Part model, mm, in its own coordinate system. Face numbers are marked on the shaded views. A direction names the side the tool comes from. Give positions to 0.01 mm unless a question says otherwise; leave off trailing zeros. Write each loop counter-clockwise with the first axis right and the second up, starting at its lowest first coordinate (ties: lowest second). Pieces come first, ordered by that corner, then holes.
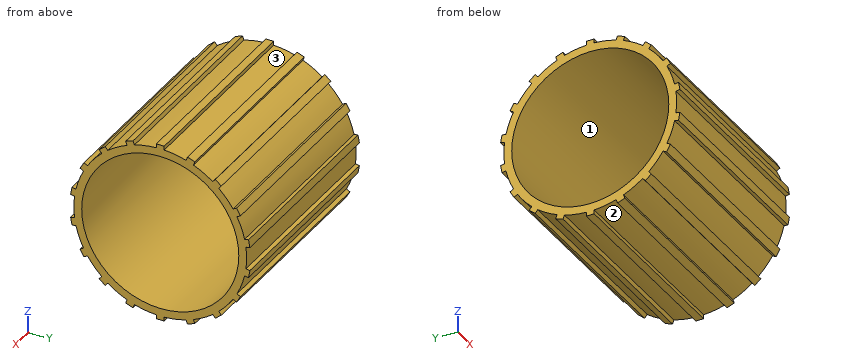
Autodesk Fusion 360 part; units mm, degrees
sketch "Sketch1" plane through (0, 0, 0) normal (0, 1, 0) x (1, 0, 0) in component "tread"
  line L0 (-50, 22) -> (0, 22)
  line L1 (0, 22) -> (0, 20)
  line L2 (0, 20) -> (-50, 20)
  line L3 (-50, 20) -> (-50, 22)
  line L4 (0, 0) -> (0, -12) construction
  dimension "d1" = 50
  dimension "d2" = 2
  dimension "d3" = 20
revolve "Revolve1" add sketch "Sketch1" angle 360 about axis through (1.75, 0, 0) along (1, 0, 0) makes body 1 in component "tread"
sketch "Sketch2" plane through (0, 0, 0) normal (0, 0, 1) x (1, 0, 0) in component "tread"
  line L0 (0, 0) -> (-50, 0)
  line L1 (0, 1) -> (-50, 1)
  line L2 (0, -1) -> (-50, -1)
  line L3 (0, -1) -> (0, 1)
  line L4 (-50, -1) -> (-50, 1)
  dimension "d5" = 50
  dimension "d6" = 1
  dimension "d7" = -1
extrude "Extrude1" add sketch "Sketch2" along normal mid plane 46 separate body makes body 2 in component "tread"
pattern_circular "C-Pattern1" count 9 over 360 about axis through (1.75, 0, 0) along (1, 0, 0) of "Extrude1" makes body 3 makes body 4 makes body 5 makes body 6 makes body 7 makes body 8 makes body 9 makes body 10 in component "tread"
sketch "Sketch3" plane through (0, 0, 0) normal (1, 0, 0) x (0, 0, -1) in component "tread"
  circle A0 centre (0, 0) radius 20
  dimension "d14" = 40
extrude "Extrude2" cut sketch "Sketch3" against normal blind 50 bodies 2 makes body 11 at (-16.6667, 1, -20.9833) in component "tread"
extrude "Extrude3" cut sketch "Sketch3" against normal blind 50 bodies 3 4 5 6 7 8 9 10 makes body 19 at (-16.6667, -13.3699, -17.4894) makes body 18 at (-33.3333, -20.4909, -4.6285) makes body 17 at (-33.3333, -18.6721, 9.6256) makes body 16 at (-16.6667, -8.4613, 20.3234) makes body 15 at (-16.6667, 6.5819, 21.0074) makes body 14 at (-16.6667, 18.5453, 11.8619) makes body 13 at (-16.6667, 21.8312, -2.834) makes body 12 at (-16.6667, 14.902, -16.2038) in component "tread"
combine "Combine1" operation add target body 1 tool bodies 5 in component "tread"
combine "Combine2" operation add target body 1 tool bodies 3 4 8 6 7 9 10 13 12 11 18 19 2 16 15 14 17 in component "tread"
component "tread" placed x (1, 0, 0) y (0, 1, 0) z (0, 0, 1) at (0, 0, 0)
1) 3-axis set-ups, long thin cutter, end or side, ignore diameter. For the marked faces 1, 2 and 3: which of +Z, -Z, +X, -X, +Y, -Y reach the whole face in a straight line?
Answers follow:
face 1: +X, -X
face 2: -Z, +X, -X
face 3: +Z, +X, -X
2) Wall check: L1, parallel to Y at x = -39, z = 0; L2, parallel to Z at x = -11, y = 0; L3, parallel to Y at x = -35.5, z = 8.5. Give the ranges that are in metal, low to high.
Answers follow:
L1: y = -22 to -20, 20 to 22
L2: z = -23 to -20, 20 to 23
L3: y = -20.29 to -18.1, 18.1 to 20.29
3) Pin check, flat tips, straight feed: pin 1 Ø1.5 at (x, z) = (-32, 4.5) entering from +Y; pin 2 Ø0.8 at (x, z) = (-26, 22.5) entering from +Y; pin 3 Ø1 at (x, z) = (-24.5, -6.5) entering from -Y. Stop position of each tip, or through.
Answers follow:
pin 1: stops at y = 22.69
pin 2: stops at y = 1
pin 3: stops at y = -21.17
4) Saw through at A-A, the plane y = 5.5. Write the cut outline in (x, z).
Answers follow:
outline: (-50, -21.3) - (0, -21.3) - (0, -19.23) - (-50, -19.23) - close; (-50, 19.23) - (0, 19.23) - (0, 21.3) - (-50, 21.3) - close
5) Saw through at B-B, the plane z = 0. Write the cut outline in (x, y), then the cut area to 3 significant figures.
Answers follow:
outline: (-50, -22) - (0, -22) - (0, -20) - (-50, -20) - close; (-50, 20) - (0, 20) - (0, 22) - (-50, 22) - close
area: 200 mm2
